Source: three-view drawing plus pictorial views. Frame: mm from the lowest corner of the part. A direction names the side the tool comes from. Give positions to 0.01 mm unless a question says otherwise; leave off trailing zeros. Loops run counter-clockwise (first coordinate to the right, second up) from the corner with the lowest first, then second, coordinate; pieces in that order, holes last. Notation, with made-up numbers: (-7, 20.25) - (-2, 20.25) arc R18 cw to (-2, 30.25) - close; hole circle Ø1 at (1, 88.25). An arc over 180 degrees is marked (long way). Answer as a JSON object with one key per item and string values. Group by question number.
(1) Pin query (flat end, axial travel): P1, Ø4, axis at x = 18, z = 15.5, coming from the +Y side; P2, Ø2, axis at x = 12, y = 4, coming from the -Z side; P3, Ø1, axis at y = 1.5, z = 6.5, coming from the +X side. Return the tip coordinate at first contact, or that it passes through.
(2) Mould query, pull axis X, two halves, no side actions, for the marked faces 1, 2, 3 and 4. Classes: +X half, -X half, draft (parallel to the pull), parting line (faces both ways), or undercut.
(3) Material intervals for L1, parallel to Z at x = 10.5, y = 0.9; L2, parallel to Z at x = 3.25, y = 0.85, sorted ascending.
(4) Section query B-B (x = 10.25). Return loops of the section in (y, z), plus the area to 3 significant figures.
(5) Section query C-C (y = 1.55). Count the separate pieces of the cut face and the enclosed holes in it, plus the area to 3 significant figures.
(6) Section query A-A (z = 10.25). Return loops of the section in (x, y), plus the area to 3 significant figures.
(7) Section query D-D (x = 7). Return loops of the section in (y, z), plus the area to 3 significant figures.
(8) Access query for the marked faces 5 and 6. Directions: +Z, -Z, +X, -X, +Y, -Y. A direction counts if a zero-diameter tool reaches every point of the face in a straight line with its end or side. Return the directions, or none.
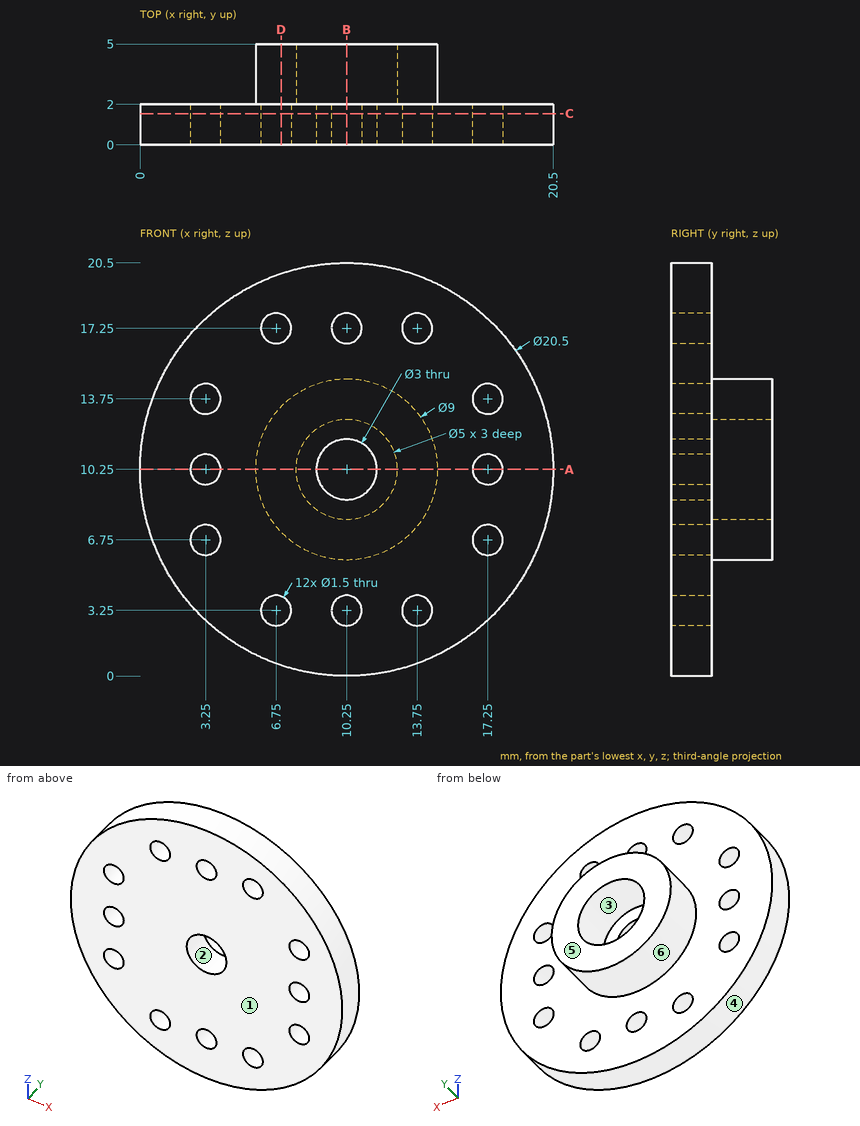
Recorded:
{
 "1": {"P1": "stops at y = 2", "P2": "stops at z = 5.81", "P3": "stops at x = 19.97"},
 "2": {"face 1": "draft", "face 2": "undercut", "face 3": "undercut", "face 4": "parting line"},
 "3": {"L1": "z = 0 to 2.54, 3.96 to 8.77, 11.73 to 16.54, 17.96 to 20.5", "L2": "z = 2.76 to 6, 7.5 to 9.5, 11 to 13, 14.5 to 17.74"},
 "4": {"outline": "(0, 0) - (2, 0) - (2, 2.5) - (0, 2.5) - close; (0, 4) - (2, 4) - (2, 5.75) - (5, 5.75) - (5, 7.75) - (2, 7.75) - (2, 8.75) - (0, 8.75) - close; (0, 11.75) - (2, 11.75) - (2, 12.75) - (5, 12.75) - (5, 14.75) - (2, 14.75) - (2, 16.5) - (0, 16.5) - close; (0, 18) - (2, 18) - (2, 20.5) - (0, 20.5) - close", "area": "41.0 mm^2"},
 "5": {"separate pieces": "1", "enclosed holes": "13", "area": "302 mm^2"},
 "6": {"outline": "(0, 0) - (2.5, 0) - (2.5, 2) - (0, 2) - close; (4, 0) - (8.75, 0) - (8.75, 2) - (7.75, 2) - (7.75, 5) - (5.75, 5) - (5.75, 2) - (4, 2) - close; (11.75, 0) - (16.5, 0) - (16.5, 2) - (14.75, 2) - (14.75, 5) - (12.75, 5) - (12.75, 2) - (11.75, 2) - close; (18, 0) - (20.5, 0) - (20.5, 2) - (18, 2) - close", "area": "41.0 mm^2"},
 "7": {"outline": "(0, 0.53) - (2, 0.53) - (2, 2.54) - (0, 2.54) - close; (0, 3.96) - (2, 3.96) - (2, 7.14) - (5, 7.14) - (5, 13.36) - (2, 13.36) - (2, 16.54) - (0, 16.54) - close; (0, 17.96) - (2, 17.96) - (2, 19.97) - (0, 19.97) - close", "area": "51.9 mm^2"},
 "8": {"face 5": "+Z, -Z, +X, -X, +Y", "face 6": "+Y"}
}
